Input: part model. Units: mm. Frame: model coordinates. A direction names the side the tool comes from. Round coordinates to 2 decimals unless told otherwise and drop trailing zeros. Loops run counter-clockwise (first coordinate to the right, second up) from the corner with the lowest first, then second, coordinate; pieces in that order, holes last. Notation, with made-up numbers: (86.5, -23) - (111.5, -23) arc R20 ccw to (111.5, 6) - close; hole circle Ø8 at (45.5, 48.5). An arc over 180 degrees is marked (long way). Write each question's results on one line, items separated by ' | '.
from build123d import *

# Parameters (mm, degrees)
SKETCH_1_W          = 55
SKETCH_1_H          = 38
EXTRUDE_1_DEPTH     = 3
SKETCH_2_R          = 10.9
EXTRUDE_2_DEPTH     = 5
SKETCH_3_R          = 4
CUT_EXTRUDE_1_DEPTH = 35.369317712
CUT_EXTRUDE_2_DEPTH = 3.6
SKETCH_5_R          = 0.5
CUT_EXTRUDE_3_DEPTH = 4
FILLET_1_R          = 5
FILLET_2_R          = 5
FILLET_3_R          = 5
FILLET_4_R          = 5
SKETCH_6_R          = 1.65
CUT_EXTRUDE_4_DEPTH = 35.369317712


with BuildPart() as part:
    # 草图1 → 凸台-拉伸1 (new body)
    with BuildSketch(Plane(origin=(0, 0, 0), x_dir=(1, 0, 0), z_dir=(0, 1, 0))):
        Rectangle(SKETCH_1_W, SKETCH_1_H)
    extrude(amount=EXTRUDE_1_DEPTH)

    # 草图2 → 凸台-拉伸2 (add)
    with BuildSketch(Plane(origin=(0, 3, 0), x_dir=(1, 0, 0), z_dir=(0, 1, 0))):
        with Locations(Location((0, 0, 0), (0, 0, 270))):
            Circle(SKETCH_2_R)
    extrude(amount=EXTRUDE_2_DEPTH)

    # 草图3 → 切除-拉伸1 (cut, through all)
    with BuildSketch(Plane.XZ):
        with Locations(Location((0, 0, 0), (0, 0, 270))):
            Circle(SKETCH_3_R)
    extrude(amount=-CUT_EXTRUDE_1_DEPTH, mode=Mode.SUBTRACT)

    # 草图4 → 切除-拉伸2 (cut)
    with BuildSketch(Plane(origin=(0, 8, 0), x_dir=(1, 0, 0), z_dir=(0, 1, 0))):
        Polygon((3.674809939, -1.579801226), (2.341337155, -12.320336373), (-2.341337155, -12.320336373), (-3.674809939, -1.579801226), align=None)
        Polygon((-3.674809939, 1.579801226), (-2.341337155, 12.320336373), (2.341337155, 12.320336373), (3.674809939, 1.579801226), align=None)
    extrude(amount=-CUT_EXTRUDE_2_DEPTH, mode=Mode.SUBTRACT)

    # 草图5 → 切除-拉伸3 (cut)
    with BuildSketch(Plane(origin=(0, 4.4, 0), x_dir=(1, 0, 0), z_dir=(0, 1, 0))):
        with Locations(Location((0, -6.5, 0), (0, 0, 270))):
            Circle(SKETCH_5_R)
        with Locations(Location((0, 6.5, 0), (0, 0, 270))):
            Circle(SKETCH_5_R)
    extrude(amount=-CUT_EXTRUDE_3_DEPTH, mode=Mode.SUBTRACT)

    # 圆角1
    fillet_1_edges = [part.edges().sort_by_distance(p)[0] for p in [
        (27.5, 1.5, 19),
    ]]
    fillet(fillet_1_edges, radius=FILLET_1_R)

    # 圆角2
    fillet_2_edges = [part.edges().sort_by_distance(p)[0] for p in [
        (-27.5, 1.5, 19),
    ]]
    fillet(fillet_2_edges, radius=FILLET_2_R)

    # 圆角3
    fillet_3_edges = [part.edges().sort_by_distance(p)[0] for p in [
        (-27.5, 1.5, -19),
    ]]
    fillet(fillet_3_edges, radius=FILLET_3_R)

    # 圆角4
    fillet_4_edges = [part.edges().sort_by_distance(p)[0] for p in [
        (27.5, 1.5, -19),
    ]]
    fillet(fillet_4_edges, radius=FILLET_4_R)

    # 草图6 → 切除-拉伸4 (cut, through all)
    with BuildSketch(Plane.XZ):
        with Locations(Location((-20, 12.5, 0), (0, 0, 270))):
            Circle(SKETCH_6_R)
        with Locations(Location((20, 12.5, 0), (0, 0, 270))):
            Circle(SKETCH_6_R)
        with Locations(Location((20, -12.5, 0), (0, 0, 270))):
            Circle(SKETCH_6_R)
        with Locations(Location((-20, -12.5, 0), (0, 0, 270))):
            Circle(SKETCH_6_R)
    extrude(amount=-CUT_EXTRUDE_4_DEPTH, mode=Mode.SUBTRACT)


solid = part.part
1. Section query C-C, the plane z = 0. Output: boundary loops of the cut face in (x, y), plus the area to 3 significant figures.
Answer:
outline: (-27.5, 0) - (-4, 0) - (-4, 8) - (-10.9, 8) - (-10.9, 3) - (-27.5, 3) - close; (4, 0) - (27.5, 0) - (27.5, 3) - (10.9, 3) - (10.9, 8) - (4, 8) - close | area: 210 mm^2
2. Mould query, pull axis X, two halves, no side actions, for faces 3 (the flat face through (0.1, 4.4, -7.3)), 4 (the cylindrical face through (-26.07, 1.52, -17.5)), 5 (the cylindrical face through (26, 1.52, -17.57)). Classes: pulls with the +X half, pulls with the -X half, needs draft (parallel to the pull), parting line crosses it, or undercut.
Answer:
face 3: undercut | face 4: pulls with the -X half | face 5: pulls with the +X half
3. Section query D-D, the plane x = 2. Output: boundary loops of the cut face in (y, z).
Answer:
outline: (0, -19) - (3, -19) - (3, -10.71) - (4.4, -10.71) - (4.4, -3.46) - (0, -3.46) - close; (0, 3.46) - (4.4, 3.46) - (4.4, 10.71) - (3, 10.71) - (3, 19) - (0, 19) - close
4. Line query: line 1 (X direction, y = 1.65, z = 12.5); line 2 (X direction, y = 2.75, z = 6.5); line 3 (X direction, y = 5.5, z = 0). Output: solid intervals per line, ascending. Write a range as [from, to].
Answer:
line 1: [-27.5, -21.65], [-18.35, 18.35], [21.65, 27.5] | line 2: [-27.5, -0.5], [0.5, 27.5] | line 3: [-10.9, -4], [4, 10.9]
5. Set-up query: faces 1 (the cylindrical face through (26, 1.52, 17.57)), 2 (the flat face through (-3.1, 6.2, 6.2)). Return all of +Z, -Z, +X, -X, +Y, -Y with unobstructed straight access to the full face (end or side cutting, diameter ignored); none if empty.
Answer:
face 1: +Z, +X, +Y, -Y | face 2: +Y
6. Contact query for flat-ended pins moving along their axis: pin 1 (1.1 mm diameter, centred on x = 0, z = -6.5, fed in from +Y); pin 2 (4.5 mm diameter, centred on x = -20, z = 12.5, fed in from +Y). Output: stop coordinate, or through.
Answer:
pin 1: y = 4.4 | pin 2: y = 3
7. Section query B-B, the plane x = -20. Output: boundary loops of the cut face in (y, z).
Answer:
outline: (0, -19) - (3, -19) - (3, -14.15) - (0, -14.15) - close; (0, -10.85) - (3, -10.85) - (3, 10.85) - (0, 10.85) - close; (0, 14.15) - (3, 14.15) - (3, 19) - (0, 19) - close
8. Section query A-A, the plane z = 12.5. Output: boundary loops of the cut face in (x, y).
Answer:
outline: (-27.5, 0) - (-21.65, 0) - (-21.65, 3) - (-27.5, 3) - close; (-18.35, 0) - (18.35, 0) - (18.35, 3) - (-18.35, 3) - close; (21.65, 0) - (27.5, 0) - (27.5, 3) - (21.65, 3) - close
